Could you check a few things on this model? Use its own coordinates, in mm. Face numbers are marked on the shaded views. A direction names the side the tool comes from. Coordinates: 2 decimals unless noted, no trailing zeros. Write each loop counter-clockwise with the first axis right and the second up, starting at its lowest first coordinate (ties: lowest second). Pieces come first, ordered by that corner, then holes. Notation, with made-up numbers: (45.5, 86) - (50.5, 86) arc R14 ccw to (50.5, 98) - close; hole circle Ø9 at (29.25, 13.5). An arc over 180 degrees is marked (long way). Answer as a JSON object with one key per item and string values. Group by question number.
1) Please list where these lines run through material, in increasing order: line 1 along X through (y, z) = (12.75, 4.25); line 2 along X through (y, z) = (11.25, 5.75); line 3 along X through (y, z) = (9.25, 2.75).
2) We'd pull the mould along X, two halves only. Please class the marked faces 1, 2 and 3: released by +X, released by -X, zero draft, split by the parting line, or undercut.
3) If we section it at B-B (x = 39): Write out the boundary of the cut face in (y, z), plus the area to 3 significant figures.
4) If we section it at D-D (y = 2.75): Write out the boundary of the cut face in (x, z), plus the area to 3 significant figures.
5) If we section it at A-A (y = 7.25): Write out the boundary of the cut face in (x, z), plus the area to 3 significant figures.
6) If we section it at C-C (z = 2.75): Write out the boundary of the cut face in (x, y) (3 decimals).
7) On a 3-axis mill with a long thin cutter (end or side, diameter ignored), from which of +Z, -Z, +X, -X, +Y, -Y can I reach the whole of each face in a straight line? I mean the marked faces 4, 5, 6 and 7. Say none if no direction works.
8) Will these pins go through, and if not, where does the flat tip stop? pin 1 Ø0.8 at (x, y) = (36.5, 12) entering from -Z; pin 2 Ø1 at (y, z) = (0.5, 1) entering from -X; pin 3 Ø2 at (x, z) = (11.5, -1.5) entering from +Y.
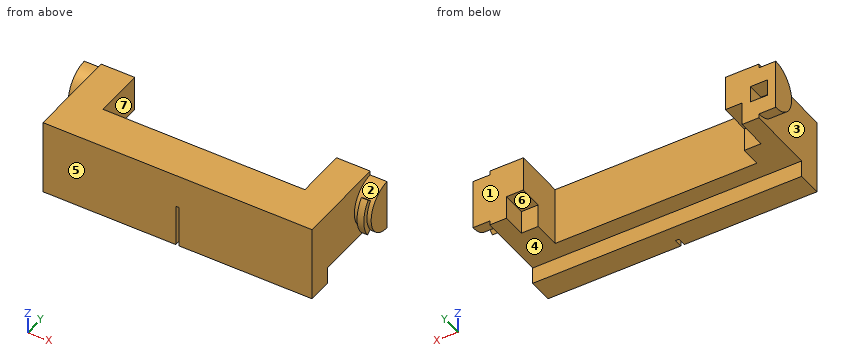
```python
from build123d import *

# Parameters (mm, degrees)
SKETCH1_W           = 40.64
SKETCH1_H           = 6.35
BOSS_EXTRUDE1_DEPTH = 8.89
SKETCH2_W           = 5.08
SKETCH2_H           = 8.89
BOSS_EXTRUDE2_DEPTH = 7.62
SKETCH3_W           = 5.08
SKETCH3_H           = 8.89
BOSS_EXTRUDE3_DEPTH = 7.62
SKETCH4_W           = 3.556
SKETCH4_H           = 4.572
CUT_EXTRUDE1_DEPTH  = 2.54
BOSS_EXTRUDE4_DEPTH = 2.54
SKETCH6_W           = 40.64
SKETCH6_H           = 3.683
BOSS_EXTRUDE5_DEPTH = 2.54
SKETCH7_W           = 3.556
SKETCH7_H           = 3.556
CUT_EXTRUDE2_DEPTH  = 2.54
BOSS_EXTRUDE6_START = 2.54
BOSS_EXTRUDE6_DEPTH = 2.54
WRAP1_SECTION_W     = 0.762
WRAP1_SECTION_H     = 1.016
WRAP1_ANGLE         = 76.394372684
SKETCH11_W          = 0.508
SKETCH11_H          = 6.35
CUT_EXTRUDE3_DEPTH  = 1.27
SKETCH12_W          = 2.54
SKETCH12_H          = 2.54
CUT_EXTRUDE4_DEPTH  = 2.54


with BuildPart() as part:
    # Sketch1 → Boss-Extrude1 (new body)
    with BuildSketch(Plane.XY):
        with Locations((20.32, 3.175)):
            Rectangle(SKETCH1_W, SKETCH1_H)
    extrude(amount=BOSS_EXTRUDE1_DEPTH)

    # Sketch2 → Boss-Extrude2 (add)
    with BuildSketch(Plane(origin=(0, 6.35, 0), x_dir=(1, 0, 0), z_dir=(0, 1, 0))):
        with Locations((2.54, -4.445)):
            Rectangle(SKETCH2_W, SKETCH2_H)
    extrude(amount=BOSS_EXTRUDE2_DEPTH)

    # Sketch3 → Boss-Extrude3 (add)
    with BuildSketch(Plane(origin=(0, 6.35, 0), x_dir=(1, 0, 0), z_dir=(0, 1, 0))):
        with Locations((38.1, -4.445)):
            Rectangle(SKETCH3_W, SKETCH3_H)
    extrude(amount=BOSS_EXTRUDE3_DEPTH)

    # Sketch4 → Cut-Extrude1 (cut)
    with BuildSketch(Plane(origin=(5.08, 0, 0), x_dir=(0, 0, -1), z_dir=(1, 0, 0))):
        with Locations((-1.778, 11.684)):
            Rectangle(SKETCH4_W, SKETCH4_H)
    extrude(amount=-CUT_EXTRUDE1_DEPTH, mode=Mode.SUBTRACT)

    # Sketch5 → Boss-Extrude4 (add)
    with BuildSketch(Plane.ZY):
        with BuildLine():
            Line((8.255, 13.97), (0.635, 13.97))
            ThreePointArc((0.635, 13.97), (4.445, 10.16), (8.255, 13.97))
        make_face()
    extrude(amount=BOSS_EXTRUDE4_DEPTH)

    # Sketch6 → Boss-Extrude5 (add)
    with BuildSketch(Plane(origin=(0, 0, 0), x_dir=(-1, 0, 0), z_dir=(0, 0, -1))):
        with Locations((-20.32, 1.8415)):
            Rectangle(SKETCH6_W, SKETCH6_H)
    extrude(amount=BOSS_EXTRUDE5_DEPTH)

    # Sketch7 → Cut-Extrude2 (cut)
    with BuildSketch(Plane.ZY.offset(-35.56)):
        with Locations((1.778, 12.192)):
            Rectangle(SKETCH7_W, SKETCH7_H)
    extrude(amount=-CUT_EXTRUDE2_DEPTH, mode=Mode.SUBTRACT)

    # Sketch8 → Boss-Extrude6 (add)
    with BuildSketch(Plane(origin=(40.64, 0, 0), x_dir=(0, 0, -1), z_dir=(1, 0, 0)).offset(BOSS_EXTRUDE6_START)):
        with BuildLine():
            Line((-0.635, 13.97), (-8.255, 13.97))
            ThreePointArc((-8.255, 13.97), (-4.445, 10.16), (-0.635, 13.97))
        make_face()
    extrude(amount=-BOSS_EXTRUDE6_DEPTH)

    # Wrap1 section (on wrap section) → Wrap1 (revolve)
    with BuildSketch(Plane(origin=(43.18, 13.97, 4.445), x_dir=(0, -0.772203868534924, 0.6353748385163658), z_dir=(0, 0.6353748385163658, 0.772203868534924))):
        with Locations((4.191, -1.143)):
            Rectangle(WRAP1_SECTION_W, WRAP1_SECTION_H)
    revolve(axis=Axis((43.18, 13.97, 4.445), (1, 0, 0)), revolution_arc=WRAP1_ANGLE)

    # Sketch11 → Cut-Extrude3 (cut)
    with BuildSketch(Plane.XZ):
        with Locations((20.32, 0.635)):
            Rectangle(SKETCH11_W, SKETCH11_H)
    extrude(amount=-CUT_EXTRUDE3_DEPTH, mode=Mode.SUBTRACT)

    # Sketch12 → Cut-Extrude4 (cut)
    with BuildSketch(Plane(origin=(0, 13.97, 0), x_dir=(1, 0, 0), z_dir=(0, 1, 0))):
        with Locations((0, -4.445)):
            Rectangle(SKETCH12_W, SKETCH12_H)
    extrude(amount=-CUT_EXTRUDE4_DEPTH, mode=Mode.SUBTRACT)


solid = part.part
```
Here are the results:
{
 "1": {"line 1": "x = -2.54 to -1.27, 1.27 to 5.08, 35.56 to 43.18", "line 2": "x = -2.54 to 5.08, 35.56 to 43.18", "line 3": "x = 0 to 5.08, 35.56 to 40.64"},
 "2": {"face 1": "zero draft", "face 2": "undercut", "face 3": "released by -X"},
 "3": {"outline": "(0, -2.54) - (3.68, -2.54) - (3.68, 0) - (13.97, 0) - (13.97, 8.89) - (0, 8.89) - close", "area": "134 mm²"},
 "4": {"outline": "(0, -2.54) - (40.64, -2.54) - (40.64, 8.89) - (0, 8.89) - close", "area": "465 mm²"},
 "5": {"outline": "(0, 0) - (5.08, 0) - (5.08, 8.89) - (0, 8.89) - close; (35.56, 0) - (40.64, 0) - (40.64, 8.89) - (35.56, 8.89) - close", "area": "90.3 mm²"},
 "6": {"outline": "(-2.54, 10.558) - (0, 10.558) - (0, 0) - (20.066, 0) - (20.066, 1.27) - (20.574, 1.27) - (20.574, 0) - (40.64, 0) - (40.64, 10.558) - (41.529, 10.558) - (41.529, 9.724) - (42.545, 9.724) - (42.545, 10.558) - (43.18, 10.558) - (43.18, 13.97) - (38.1, 13.97) - (38.1, 10.414) - (35.56, 10.414) - (35.56, 6.35) - (5.08, 6.35) - (5.08, 9.398) - (2.54, 9.398) - (2.54, 13.97) - (-2.54, 13.97) - close"},
 "7": {"face 4": "-Z, +X, -X, +Y", "face 5": "+Z, -Z, +X, -X, -Y", "face 6": "-Z, +Y", "face 7": "+Z, -Z, +Y"},
 "8": {"pin 1": "stops at z = 3.56", "pin 2": "stops at x = 0", "pin 3": "stops at y = 3.68"}
}
